Could you check a few things on this model? Use its own coordinates, in mm. Give positions to 0.01 mm unless a question says otherwise; leave off trailing zeros. Order: outer loops, then holes, each group sorted by start corner. A loop starts at its lowest first (then second) coordinate and runs counter-clockwise, first axis right, second up. Notation, with made-up numbers: (51, 46.25) - (58, 46.25) arc R12 ccw to (58, 54.25) - close; hole circle Ø5 at (32.25, 23.25). An arc over 180 degrees is marked (long way). One line per question, with ' | ' between items. Start each with the question number.
1. Imagine slicing it at B-B (x = 0.5). Please give me the cut outline in (y, z).
2. I need wall thicknesses on probe 1 along Y at (x, z) = (2, 0.3); probe 2 along X at (y, z) = (-0.5, 0.4); probe 3 along Y at (x, z) = (-30, 0.5). Which ranges of each line are inside material? Lowest first, please. Write a range as from..to.
3. Imagine slicing it at D-D (y = -4.5). Please give me the cut outline in (x, z).
4. For P1, Ø3, axis at x = -30.97, y = 0, coming from the +Z side, with a flat end and sliding along its axis, tell me the tip position at first contact or that it passes through.
5. Imagine slicing it at A-A (y = 0). Please give me the cut outline in (x, z).
6. Imagine slicing it at C-C (z = 1). Please give me the cut outline in (x, y).
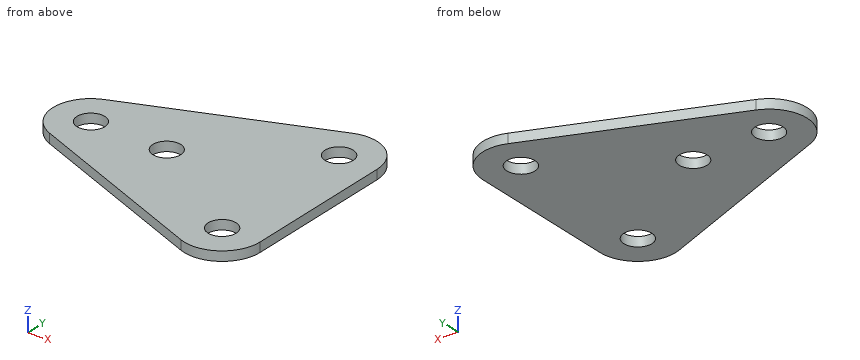
Autodesk Inventor part; units mm, degrees
ref_plane "YZ Plane" through (0, 0, 0) normal (1, 0, 0) x (0, 1, 0)
ref_plane "XZ Plane" through (0, 0, 0) normal (0, 1, 0) x (-1, 0, 0)
ref_plane "XY Plane" through (0, 0, 0) normal (0, 0, 1) x (1, 0, 0)
sketch "Sketch1" plane through (0, 0, 0) normal (0, 0, 1) x (1, 0, 0)
  circle A0 centre (0.7751, 12.7) radius 2.1844 construction
  circle A1 centre (0.7751, -12.7) radius 2.1844 construction
  circle A2 centre (0.7751, 12.7) radius 2.3495
  circle A3 centre (0.7751, -12.7) radius 2.3495
  circle A4 centre (-18.2749, 0) radius 2.3368
  circle A5 centre (-30.9749, 0) radius 2.3368
  circle A6 centre (-30.9749, 0) radius 6.35
  circle A7 centre (0.7751, -12.7) radius 6.35
  circle A8 centre (0.7751, 12.7) radius 6.35
  line L0 (7.1251, 12.7) -> (7.1251, -12.7)
  line L1 (-1.5832, -18.5958) -> (-33.3332, -5.8958)
  line L2 (-1.5832, 18.5958) -> (-33.3332, 5.8958)
  point P0 (0, 0)
  dimension "d0" = 4.699
  dimension "d1" = 4.699
  dimension "d2" = 4.6736
  dimension "d3" = 4.6736
  dimension "d4" = 12.7
  dimension "d5" = 19.05
  dimension "d6" = 12.7
  dimension "d7" = 12.7
  dimension "d8" = 12.7
extrude "Plate1" add sketch "Sketch1" along normal blind 1.5875 contours A6 | A6 L2 A8 L0 A7 L1
sheet face with bend "Face2" sketch "Sketch1" thickness 1.5875 toward (0, 0, 1) bend radius 1.5875 contours A8 | A7
bend "Bend1"
equation "\"d9\" = Thickness"
equation "\"d10\" = BendRadius"
equation "\"d11\" = BendReliefWidth"
equation "\"d13\" = MinimumRemnant"
equation "\"d12\" = BendReliefDepth"
equation "\"d14\" = TransitionRadius"
equation "\"BendRadius\" = Thickness"
equation "\"BendReliefWidth\" = Thickness"
equation "\"BendReliefDepth\" = 0.5 * Thickness"
equation "\"CornerReliefSize\" = 4 * Thickness"
equation "\"MinimumRemnant\" = 2 * Thickness"
equation "\"TransitionRadius\" = BendRadius"
equation "\"JacobiRadiusSize\" = BendRadius"
equation "\"GapSize\" = Thickness"
properties part number "imuMount"
Results found:
1) outline: (-19.04, 0) - (-15.03, 0) - (-15.03, 1.59) - (-19.04, 1.59) - close; (-10.37, 0) - (10.37, 0) - (10.37, 1.59) - (-10.37, 1.59) - close; (15.03, 0) - (19.04, 0) - (19.04, 1.59) - (15.03, 1.59) - close
2) probe 1: y = -18.93..-14.7, -10.7..10.7, 14.7..18.93 | probe 2: x = -37.31..-33.26, -28.69..-20.56, -15.99..7.13 | probe 3: y = -7.23..-2.12, 2.12..7.23
3) outline: (-35.46, 0) - (7.13, 0) - (7.13, 1.59) - (-35.46, 1.59) - close
4) P1: passes through
5) outline: (-37.32, 0) - (-33.31, 0) - (-33.31, 1.59) - (-37.32, 1.59) - close; (-28.64, 0) - (-20.61, 0) - (-20.61, 1.59) - (-28.64, 1.59) - close; (-15.94, 0) - (7.13, 0) - (7.13, 1.59) - (-15.94, 1.59) - close
6) outline: (-33.33, -5.9) - (-1.58, -18.6) arc R6.35 ccw to (7.13, -12.7) - (7.13, 12.7) arc R6.35 ccw to (-1.58, 18.6) - (-33.33, 5.9) arc R6.35 ccw to start; hole circle Ø4.67 at (-30.97, 0); hole circle Ø4.67 at (-18.27, 0); hole circle Ø4.7 at (0.78, -12.7); hole circle Ø4.7 at (0.78, 12.7)
